from build123d import *

# Parameters (mm, degrees)
SKETCH1_W                       = 106.27
SKETCH1_H                       = 122
BOSS_EXTRUDE1_DEPTH             = 73.8
SKETCH2_W                       = 86.27
SKETCH2_H                       = 102
CUT_EXTRUDE1_DEPTH              = 68.8
FILLET1_R                       = 10
FILLET2_R                       = 10
FILLET3_R                       = 7.5
FILLET4_R                       = 7.5
FILLET6_R                       = 5
SKETCH3_R                       = 3.04
CUT_EXTRUDE2_DEPTH              = 5
SKETCH4_R                       = 10.75
CUT_EXTRUDE3_DEPTH              = 5
SKETCH5_R                       = 2.5
CUT_EXTRUDE4_DEPTH              = 5
F_4_40_TAPPED_HOLE3_D           = 2.2606
F_4_40_TAPPED_HOLE3_DEPTH       = 30
F_4_40_TAPPED_HOLE3_CSINK_D     = 4.1148
F_4_40_TAPPED_HOLE3_CSINK_ANGLE = 100
F_4_40_TAPPED_HOLE3_TIP         = 0.679152758
F_4_40_TAPPED_HOLE4_D           = 2.2606
F_4_40_TAPPED_HOLE4_DEPTH       = 30
F_4_40_TAPPED_HOLE4_CSINK_D     = 4.1148
F_4_40_TAPPED_HOLE4_CSINK_ANGLE = 100
F_4_40_TAPPED_HOLE4_TIP         = 0.679152758


with BuildPart() as part:
    # Sketch1 → Boss-Extrude1 (new body)
    with BuildSketch(Plane(origin=(0, 0, 0), x_dir=(1, 0, 0), z_dir=(0, 1, 0))):
        Rectangle(SKETCH1_W, SKETCH1_H)
    extrude(amount=BOSS_EXTRUDE1_DEPTH)

    # Sketch2 → Cut-Extrude1 (cut)
    with BuildSketch(Plane.XZ):
        Rectangle(SKETCH2_W, SKETCH2_H)
    extrude(amount=-CUT_EXTRUDE1_DEPTH, mode=Mode.SUBTRACT)

    # Fillet1
    fillet1_edges = [part.edges().sort_by_distance(p)[0] for p in [
        (-53.135, 73.8, 0),
        (0, 73.8, 61),
        (53.135, 73.8, 0),
        (0, 73.8, -61),
    ]]
    fillet(fillet1_edges, radius=FILLET1_R)

    # Fillet2
    # the kernel refuses this fillet: 10 mm, written as the material it takes off along each edge
    with BuildSketch(Plane(origin=(43.135, 63.8, 51), x_dir=(1, 0, 0), z_dir=(0, 0, 1))) as fillet2_piece_1_section:
        Polygon((0, 0), (FILLET2_R, 0), (FILLET2_R, FILLET2_R), (0, FILLET2_R), align=None)
    fillet2_piece_1 = extrude(amount=FILLET2_R, mode=Mode.PRIVATE)
    fillet2_piece_1 = fillet2_piece_1 - Plane(origin=(43.135, 63.8, 51), x_dir=(-0.7071067811865475, -0.7071067811865475, 0), z_dir=(0, 0, 1)) * Sphere(FILLET2_R, mode=Mode.PRIVATE)
    add(fillet2_piece_1, mode=Mode.SUBTRACT)
    with BuildSketch(Plane(origin=(-43.135, 63.8, 51), x_dir=(-1, 0, 0), z_dir=(0, 0, 1))) as fillet2_piece_2_section:
        Polygon((0, 0), (FILLET2_R, 0), (FILLET2_R, -FILLET2_R), (0, -FILLET2_R), align=None)
    fillet2_piece_2 = extrude(amount=FILLET2_R, mode=Mode.PRIVATE)
    fillet2_piece_2 = fillet2_piece_2 - Plane(origin=(-43.135, 63.8, 51), x_dir=(0.7071067811865475, -0.7071067811865475, 0), z_dir=(0, 0, 1)) * Sphere(FILLET2_R, mode=Mode.PRIVATE)
    add(fillet2_piece_2, mode=Mode.SUBTRACT)
    with BuildSketch(Plane(origin=(43.135, 63.8, -51), x_dir=(0, 0, -1), z_dir=(1, 0, 0))) as fillet2_piece_3_section:
        Polygon((0, 0), (FILLET2_R, 0), (FILLET2_R, FILLET2_R), (0, FILLET2_R), align=None)
    fillet2_piece_3 = extrude(amount=FILLET2_R, mode=Mode.PRIVATE)
    fillet2_piece_3 = fillet2_piece_3 - Plane(origin=(43.135, 63.8, -51), x_dir=(0, -0.7071067811865475, 0.7071067811865475), z_dir=(1, 0, 0)) * Sphere(FILLET2_R, mode=Mode.PRIVATE)
    add(fillet2_piece_3, mode=Mode.SUBTRACT)
    with BuildSketch(Plane(origin=(-43.135, 63.8, -51), x_dir=(0, 0, -1), z_dir=(-1, 0, 0))) as fillet2_piece_4_section:
        Polygon((0, 0), (FILLET2_R, 0), (FILLET2_R, -FILLET2_R), (0, -FILLET2_R), align=None)
    fillet2_piece_4 = extrude(amount=FILLET2_R, mode=Mode.PRIVATE)
    fillet2_piece_4 = fillet2_piece_4 - Plane(origin=(-43.135, 63.8, -51), x_dir=(0, -0.7071067811865475, 0.7071067811865475), z_dir=(-1, 0, 0)) * Sphere(FILLET2_R, mode=Mode.PRIVATE)
    add(fillet2_piece_4, mode=Mode.SUBTRACT)
    with BuildSketch(Plane(origin=(-53.135, -25, -61), x_dir=(0, 0, 1), z_dir=(0, 1, 0)), Plane(origin=(-53.135, -25, 61), x_dir=(1, 0, 0), z_dir=(0, 1, 0))) as fillet2_piece_5:
        with BuildLine():
            CenterArc((FILLET2_R, FILLET2_R), FILLET2_R, 180, 90)
            Line((0, FILLET2_R), (0, 0))
            Line((0, 0), (FILLET2_R, 0))
        make_face()
    extrude(amount=88.8, mode=Mode.SUBTRACT)
    with BuildSketch(Plane(origin=(53.135, -25, -61), x_dir=(0, 0, 1), z_dir=(0, 1, 0)), Plane(origin=(53.135, -25, 61), x_dir=(-1, 0, 0), z_dir=(0, 1, 0))) as fillet2_piece_6:
        with BuildLine():
            CenterArc((FILLET2_R, -FILLET2_R), FILLET2_R, 90, 90)
            Line((0, -FILLET2_R), (0, 0))
            Line((0, 0), (FILLET2_R, 0))
        make_face()
    extrude(amount=88.8, mode=Mode.SUBTRACT)

    # Fillet3
    fillet3_edges = [part.edges().sort_by_distance(p)[0] for p in [
        (43.135, 68.8, 0),
        (0, 68.8, -51),
        (-43.135, 68.8, 0),
        (0, 68.8, 51),
    ]]
    fillet(fillet3_edges, radius=FILLET3_R)

    # Fillet4
    # the kernel refuses this fillet: 7.5 mm, written as the material it adds along each edge
    with BuildSketch(Plane(origin=(-35.635, 61.3, -43.5), x_dir=(0, 0, -1), z_dir=(-1, 0, 0))) as fillet4_piece_1_section:
        Polygon((0, 0), (FILLET4_R, 0), (FILLET4_R, -FILLET4_R), (0, -FILLET4_R), align=None)
    fillet4_piece_1 = extrude(amount=FILLET4_R, mode=Mode.PRIVATE)
    fillet4_piece_1 = fillet4_piece_1 - Plane(origin=(-35.635, 61.3, -43.5), x_dir=(0, -0.7071067811865475, 0.7071067811865475), z_dir=(-1, 0, 0)) * Sphere(FILLET4_R, mode=Mode.PRIVATE)
    add(fillet4_piece_1)
    with BuildSketch(Plane(origin=(-35.635, 61.3, 43.5), x_dir=(0, 0, 1), z_dir=(-1, 0, 0))) as fillet4_piece_2_section:
        Polygon((0, 0), (FILLET4_R, 0), (FILLET4_R, FILLET4_R), (0, FILLET4_R), align=None)
    fillet4_piece_2 = extrude(amount=FILLET4_R, mode=Mode.PRIVATE)
    fillet4_piece_2 = fillet4_piece_2 - Plane(origin=(-35.635, 61.3, 43.5), x_dir=(0, -0.7071067811865475, -0.7071067811865475), z_dir=(-1, 0, 0)) * Sphere(FILLET4_R, mode=Mode.PRIVATE)
    add(fillet4_piece_2)
    with BuildSketch(Plane(origin=(35.635, 61.3, -43.5), x_dir=(1, 0, 0), z_dir=(0, 0, -1))) as fillet4_piece_3_section:
        Polygon((0, 0), (FILLET4_R, 0), (FILLET4_R, -FILLET4_R), (0, -FILLET4_R), align=None)
    fillet4_piece_3 = extrude(amount=FILLET4_R, mode=Mode.PRIVATE)
    fillet4_piece_3 = fillet4_piece_3 - Plane(origin=(35.635, 61.3, -43.5), x_dir=(-0.7071067811865475, -0.7071067811865475, 0), z_dir=(0, 0, -1)) * Sphere(FILLET4_R, mode=Mode.PRIVATE)
    add(fillet4_piece_3)
    with BuildSketch(Plane(origin=(35.635, 61.3, 43.5), x_dir=(1, 0, 0), z_dir=(0, 0, 1))) as fillet4_piece_4_section:
        Polygon((0, 0), (FILLET4_R, 0), (FILLET4_R, FILLET4_R), (0, FILLET4_R), align=None)
    fillet4_piece_4 = extrude(amount=FILLET4_R, mode=Mode.PRIVATE)
    fillet4_piece_4 = fillet4_piece_4 - Plane(origin=(35.635, 61.3, 43.5), x_dir=(-0.7071067811865475, -0.7071067811865475, 0), z_dir=(0, 0, 1)) * Sphere(FILLET4_R, mode=Mode.PRIVATE)
    add(fillet4_piece_4)
    with BuildSketch(Plane(origin=(43.135, 0, 51), x_dir=(-1, 0, 0), z_dir=(0, 1, 0)), Plane(origin=(-43.135, 0, 51), x_dir=(0, 0, -1), z_dir=(0, 1, 0))) as fillet4_piece_5:
        with BuildLine():
            CenterArc((FILLET4_R, -FILLET4_R), FILLET4_R, 90, 90)
            Line((0, -FILLET4_R), (0, 0))
            Line((0, 0), (FILLET4_R, 0))
        make_face()
    extrude(amount=61.3)
    with BuildSketch(Plane(origin=(43.135, 0, -51), x_dir=(-1, 0, 0), z_dir=(0, 1, 0)), Plane(origin=(-43.135, 0, -51), x_dir=(0, 0, 1), z_dir=(0, 1, 0))) as fillet4_piece_6:
        with BuildLine():
            CenterArc((FILLET4_R, FILLET4_R), FILLET4_R, 180, 90)
            Line((0, FILLET4_R), (0, 0))
            Line((0, 0), (FILLET4_R, 0))
        make_face()
    extrude(amount=61.3)

    # Fillet6
    fillet6_edges = [part.edges().sort_by_distance(p)[0] for p in [
        (-53.135, 0, 0),
        (53.135, 0, 0),
        (0, 0, 61),
        (0, 0, -61),
        (-50.206067812, 0, 58.071067812),
        (50.206067812, 0, 58.071067812),
        (50.206067812, 0, -58.071067812),
        (-50.206067812, 0, -58.071067812),
    ]]
    fillet(fillet6_edges, radius=FILLET6_R)

    # Sketch3 → Cut-Extrude2 (cut)
    with BuildSketch(Plane(origin=(0, 73.8, 0), x_dir=(1, 0, 0), z_dir=(0, 1, 0))):
        with Locations(Location((14.265, -16, 0), (0, 0, 270))):
            Circle(SKETCH3_R)
        with Locations(Location((6.765, -16, 0), (0, 0, 270))):
            Circle(SKETCH3_R)
    extrude(amount=-CUT_EXTRUDE2_DEPTH, mode=Mode.SUBTRACT)

    # Sketch4 → Cut-Extrude3 (cut)
    with BuildSketch(Plane(origin=(0, 73.8, 0), x_dir=(1, 0, 0), z_dir=(0, 1, 0))):
        with Locations(Location((-23.135, -31, 0), (0, 0, 270))):
            Circle(SKETCH4_R)
    extrude(amount=-CUT_EXTRUDE3_DEPTH, mode=Mode.SUBTRACT)

    # Sketch5 → Cut-Extrude4 (cut)
    with BuildSketch(Plane(origin=(0, 73.8, 0), x_dir=(1, 0, 0), z_dir=(0, 1, 0))):
        with Locations(Location((4.865, -25.3, 0), (0, 0, 270))):
            Circle(SKETCH5_R)
        with Locations(Location((12.865, -25.3, 0), (0, 0, 270))):
            Circle(SKETCH5_R)
    extrude(amount=-CUT_EXTRUDE4_DEPTH, mode=Mode.SUBTRACT)

    # #4-40 Tapped Hole3
    with Locations(Plane(origin=(100.412065725, -2, -32.702388863), x_dir=(-1, 0, 0), z_dir=(0, -1, 0))):
        with Locations((143.547065725, -83.702388863)):
            CounterSinkHole(F_4_40_TAPPED_HOLE3_D / 2, F_4_40_TAPPED_HOLE3_CSINK_D / 2, depth=F_4_40_TAPPED_HOLE3_DEPTH, counter_sink_angle=F_4_40_TAPPED_HOLE3_CSINK_ANGLE)
            with Locations((0, 0, -(F_4_40_TAPPED_HOLE3_DEPTH + F_4_40_TAPPED_HOLE3_TIP / 2))):  # 118° drill point
                Cone(0, F_4_40_TAPPED_HOLE3_D / 2, F_4_40_TAPPED_HOLE3_TIP, mode=Mode.SUBTRACT)

    # #4-40 Tapped Hole4
    with Locations(Plane(origin=(100.412065725, -2, -32.702388863), x_dir=(-1, 0, 0), z_dir=(0, -1, 0))):
        with Locations((57.277065725, 18.297611137)):
            CounterSinkHole(F_4_40_TAPPED_HOLE4_D / 2, F_4_40_TAPPED_HOLE4_CSINK_D / 2, depth=F_4_40_TAPPED_HOLE4_DEPTH, counter_sink_angle=F_4_40_TAPPED_HOLE4_CSINK_ANGLE)
            with Locations((0, 0, -(F_4_40_TAPPED_HOLE4_DEPTH + F_4_40_TAPPED_HOLE4_TIP / 2))):  # 118° drill point
                Cone(0, F_4_40_TAPPED_HOLE4_D / 2, F_4_40_TAPPED_HOLE4_TIP, mode=Mode.SUBTRACT)


solid = part.part
Here's how the part is built. I have some questions about the finished solid (model axes, mm). A direction names the side the tool comes from. Coordinates: 2 decimals unless noted, no trailing zeros. Write each loop counter-clockwise with the first axis right and the second up, starting at its lowest first coordinate (ties: lowest second). Pieces come first, ordered by that corner, then holes.
Item 1: If we mould it in two halves opening along Z, with no side actions, what happens to faces 1 (the cylindrical face through (40.88, 30.22, 48.86)), 2 (the flat face through (-47, 0, 0)), 3 (the cylindrical face through (50.128, 33.988, 58.148)), 4 (the cylindrical face through (-41, 66.54, 0.61))? For each: +Z half, -Z half, draft (parallel to the pull), parting line (faces both ways), or undercut.
Item 2: If I drill on line 1 (X direction, y = 70, z = 16) (3 decimals); line 2 (X direction, y = 28.5, z = 19.5) (3 decimals); line 3 (Z direction, x = -15.5, y = 13.5), over which ranges is the centre line in solid material (lowest first)?
Item 3: I want a section at C-C on y = 34. Write out the boundary of the cut face in (x, z) (3 decimals).
Item 4: I want a section at A-A on y = 21.5. Write out the boundary of the cut face in (x, z) (3 decimals).
Item 5: On a 3-axis mill with a long thin cutter (end or side, diameter ignored), from which of +Z, -Z, +X, -X, +Y, -Y can I reach the whole of each face in a straight line? I mean faces 5 (the flat face through (-1, 34, 61)), 6 (the flat face through (0, 30, 51)). Say none if no direction works.
Item 6: I want a section at B-B on z = 16. Write out the boundary of the cut face in (x, y) (3 decimals).
Item 7: Will these pins go through, and if not, where does the flat tip stop? pin 1 (9.5 mm diameter, centred on x = 14.265, z = 16, fed in from -Y); pin 2 (3 mm diameter, centred on x = 4.865, z = 25.3, fed in from +Y); pin 3 (4 mm diameter, centred on x = 25.5, y = 66, fed in from -Z); pin 4 (1.4 mm diameter, centred on x = -43.135, z = 51, fed in from -Y).
Item 8: I want a section at D-D on x = -28.5. Write out the boundary of the cut face in (y, z).
Findings below:
1. face 1: undercut
1. face 2: draft
1. face 3: +Z half
1. face 4: undercut
2. line 1: x = -50.981 to 3.725, 9.805 to 11.225, 17.305 to 50.981
2. line 2: x = -53.135 to -43.135, 43.135 to 53.135
2. line 3: z = -61 to -51, 51 to 61
3. outline: (-53.135, -51) arc R10 ccw to (-43.135, -61) - (43.135, -61) arc R10 ccw to (53.135, -51) - (53.135, 51) arc R10 ccw to (43.135, 61) - (-43.135, 61) arc R10 ccw to (-53.135, 51) - close; hole (-43.135, -43.5) arc R7.5 ccw to (-35.635, -51) - (35.635, -51) arc R7.5 ccw to (43.135, -43.5) - (43.135, 43.5) arc R7.5 ccw to (35.635, 51) - (-35.635, 51) arc R7.5 ccw to (-43.135, 43.5) - close
4. outline: (-53.135, -51) arc R10 ccw to (-43.135, -61) - (43.135, -61) arc R10 ccw to (53.135, -51) - (53.135, 51) arc R10 ccw to (43.135, 61) - (-43.135, 61) arc R10 ccw to (-53.135, 51) - close; hole circle Ø2.261 at (-43.135, 51); hole (-43.135, -43.5) arc R7.5 ccw to (-35.635, -51) - (35.635, -51) arc R7.5 ccw to (43.135, -43.5) - (43.135, 43.5) arc R7.5 ccw to (35.635, 51) - (-35.635, 51) arc R7.5 ccw to (-43.135, 43.5) - close; hole circle Ø2.261 at (43.135, -51)
5. face 5: +Z, +X, -X, +Y, -Y
5. face 6: -Y
6. outline: (-53.135, 5) arc R5 ccw to (-48.135, 0) - (-43.135, 0) - (-43.135, 61.3) arc R7.5 cw to (-35.635, 68.8) - (3.725, 68.8) - (3.725, 73.8) - (-43.135, 73.8) arc R10 ccw to (-53.135, 63.8) - close; (9.805, 68.8) - (11.225, 68.8) - (11.225, 73.8) - (9.805, 73.8) - close; (17.305, 68.8) - (35.635, 68.8) arc R7.5 cw to (43.135, 61.3) - (43.135, 0) - (48.135, 0) arc R5 ccw to (53.135, 5) - (53.135, 63.8) arc R10 ccw to (43.135, 73.8) - (17.305, 73.8) - close
7. pin 1: stops at y = 68.8
7. pin 2: passes through
7. pin 3: stops at z = -61
7. pin 4: stops at y = 28.26
8. outline: (0, -56) arc R5 ccw to (5, -61) - (63.8, -61) arc R10 ccw to (73.8, -51) - (73.8, 21.68) - (68.8, 21.68) - (68.8, -43.5) arc R7.5 cw to (61.3, -51) - (0, -51) - close; (0, 51) - (61.3, 51) arc R7.5 cw to (68.8, 43.5) - (68.8, 40.32) - (73.8, 40.32) - (73.8, 51) arc R10 ccw to (63.8, 61) - (5, 61) arc R5 ccw to (0, 56) - close
